Input: part model. Units: mm. Frame: model coordinates. Face numbers are marked on the shaded views. A direction names the side the tool comes from. Give positions to 0.01 mm unless a question says otherwise; leave off trailing zeros. Loops run counter-clockwise (first coordinate to the right, second up) from the corner with the lowest first, then second, coordinate; pieces in that order, holes last. Notation, with made-up numbers: M 89,-1 L 119,-1 A24 cw 119,16 Z; hole C 89.5,-35 d5. An arc over 180 degrees is marked long. One line per item, written item: value. Start each with the question number.
(1) Pin query (flat end, axial travel): P1, Ø14, axis at x = 84.5, y = 11.5, coming from the -Z side; P2, Ø6, axis at y = 27.5, z = 4.5, coming from the -X side; P3, Ø7, axis at x = 60, y = 40, coming from the +Z side; P4, Ø10.5, axis at x = 60, y = 40, coming from the +Z side. Return the tip coordinate at first contact, or that it passes through.
(2) Access query for the marked faces 4 and 5. Directions: +Z, -Z, +X, -X, +Y, -Y. A direction counts if a zero-diameter tool reaches every point of the face in a straight line with its end or side. Return the directions, or none.
(3) Section B-B on x = 120. Output: boundary loops of the cut face in (y, z), plus the area to 3 significant figures.
(4) Section D-D on x = 1. Output: boundary loops of the cut face in (y, z).
(5) Section A-A on y = 0. Output: boundary loops of the cut face in (x, z).
(6) Pull-direction query (X, two-part tool) for the marked faces 1, 2 and 3; classes: released by +X, released by -X, zero draft, split by the parting line, or undercut.
(7) Ray query, line 1 along Y through (x, z) = (60, 17.05); line 2 along Y through (x, z) = (120, 17); line 3 along X through (y, z) = (-1, 16.75). Return the intervals inside material, ascending. Write a range as from..to.
(8) Section C-C on y = 40. Output: boundary loops of the cut face in (x, z).
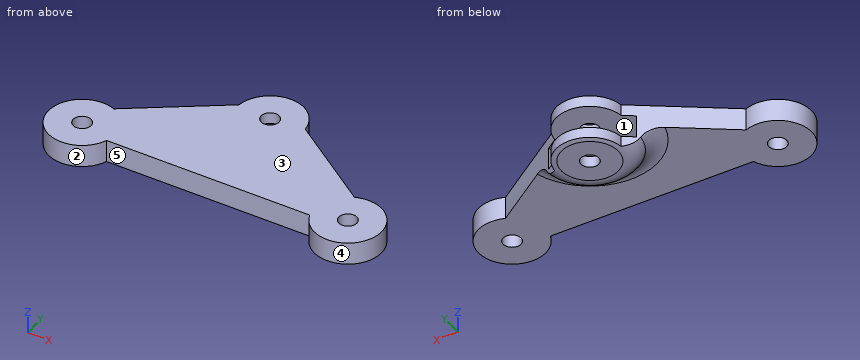
```python
from build123d import *

# Parameters (mm, degrees)
SKETCH1_R               = 4
BOSS_EXTRUDE1_DEPTH     = 20
SKETCH2_R               = 4
CUT_EXTRUDE1_DEPTH      = 10
FILLET2_R               = 10
CUT_EXTRUDE2_DEPTH      = 5
CUT_EXTRUDE2_DEPTH_BACK = 5
SKETCH5_R               = 20


with BuildPart() as part:
    # Sketch1 → Boss-Extrude1 (new body)
    with BuildSketch(Plane.XY):
        with BuildLine():
            Line((5.660747058, 13.890858244), (45.074020085, 41.488329122))
            ThreePointArc((45.074020085, 41.488329122), (60, 55), (74.925979915, 41.488329122))
            Line((74.925979915, 41.488329122), (114.339252942, 13.890858244))
            ThreePointArc((114.339252942, 13.890858244), (133.684102891, -6.143722656), (105.857864376, -5))
            Line((105.857864376, -5), (14.142135624, -5))
            ThreePointArc((14.142135624, -5), (-13.684102891, -6.143722656), (5.660747058, 13.890858244))
        make_face()
        with Locations((60, 40)):
            Circle(SKETCH1_R, mode=Mode.SUBTRACT)
        with Locations((120, 0)):
            Circle(SKETCH1_R, mode=Mode.SUBTRACT)
        Circle(SKETCH1_R, mode=Mode.SUBTRACT)
    extrude(amount=BOSS_EXTRUDE1_DEPTH)

    # Sketch2 → Cut-Extrude1 (cut)
    with BuildSketch(Plane(origin=(0, 0, 0), x_dir=(-1, 0, 0), z_dir=(0, 0, -1))):
        with BuildLine():
            ThreePointArc((-40.099720592, 38.00528712), (-60, 20), (-79.900279408, 38.00528712))
            Line((-79.900279408, 38.00528712), (-114.339252942, 13.890858244))
            ThreePointArc((-114.339252942, 13.890858244), (-133.684102891, -6.143722656), (-105.857864376, -5))
            Line((-105.857864376, -5), (-14.142135624, -5))
            ThreePointArc((-14.142135624, -5), (13.684102891, -6.143722656), (-5.660747058, 13.890858244))
            Line((-5.660747058, 13.890858244), (-40.099720592, 38.00528712))
        make_face()
        with Locations((-120, 0)):
            Circle(SKETCH2_R, mode=Mode.SUBTRACT)
        Circle(SKETCH2_R, mode=Mode.SUBTRACT)
    extrude(amount=-CUT_EXTRUDE1_DEPTH, mode=Mode.SUBTRACT)

    # Fillet2
    fillet2_edges = [part.edges().sort_by_distance(p)[0] for p in [
        (60, 20, 10),
    ]]
    fillet(fillet2_edges, radius=FILLET2_R - 0.0001)  # a hair under: the kernel refuses the full size

    # Fillet3: read off the stored shape, not the designer's step
    # Fillet3 outline → Fillet3 (revolve, cut)
    with BuildSketch(Plane(origin=(60, 40, 0), x_dir=(1, 0, 0), z_dir=(0, -1, 0))):
        with BuildLine():
            Line((21.33974599, 0), (21.33974599, 5.000000048))
            ThreePointArc((21.33974599, 5.000000048), (17.679491948, 1.339745976), (12.679491924, 0))
            Line((12.679491924, 0), (21.33974599, 0))
        make_face()
    revolve(axis=Axis((60, 40, 0), (0, 0, 1)), mode=Mode.SUBTRACT)

    # Sketch5 → Cut-Extrude2 (cut, two sides: drawn at the far end of the back side and taken through both)
    with BuildSketch(Plane.XY.offset(10).offset(-CUT_EXTRUDE2_DEPTH_BACK)):
        with Locations((60, 40)):
            Circle(SKETCH5_R)
    extrude(amount=CUT_EXTRUDE2_DEPTH + CUT_EXTRUDE2_DEPTH_BACK, mode=Mode.SUBTRACT)


solid = part.part
```
Output values:
1. P1: stops at z = 10
1. P2: stops at x = 39.84
1. P3: passes through
1. P4: stops at z = 20
2. face 4: +Z, -Z
2. face 5: +Z, -Z, -Y
3. outline: M -15,10 L -4,10 L -4,20 L -15,20 Z; M 4,10 L 15,10 L 15,20 L 4,20 Z
3. area: 220 mm²
4. outline: M -14.97,10 L -3.87,10 L -3.87,20 L -14.97,20 Z; M 3.87,10 L 14.97,10 L 14.97,20 L 3.87,20 Z
5. outline: M -15,10 L -4,10 L -4,20 L -15,20 Z; M 4,10 L 116,10 L 116,20 L 4,20 Z; M 124,10 L 135,10 L 135,20 L 124,20 Z
6. face 1: undercut
6. face 2: undercut
6. face 3: zero draft
7. line 1: y = -5..36, 44..55
7. line 2: y = -15..-4, 4..15
7. line 3: x = -14.97..-3.87, 3.87..116.13, 123.87..134.97
8. outline: M 42.95,1.01 A10 ccw 47.32,0 L 56,0 L 56,5 L 42.95,5 Z; M 42.95,15 L 56,15 L 56,20 L 42.95,20 Z; M 64,0 L 72.68,0 A10 ccw 77.05,1.01 L 77.05,5 L 64,5 Z; M 64,15 L 77.05,15 L 77.05,20 L 64,20 Z
